Model file for the job. Use its own axes, mm. Face numbers are marked on the shaded views. A direction names the side the tool comes from. Give positions to 0.01 mm unless a question says otherwise; leave off trailing zeros. Loops run counter-clockwise (first coordinate to the right, second up) from the corner with the lowest first, then second, coordinate; pieces in that order, holes last. Notation, with made-up numbers: (33.25, -5.5) - (80.25, -5.5) arc R19 cw to (80.25, 17.5) - close; hole circle Ø3 at (37.5, -34.5). An arc over 180 degrees is marked (long way). Use a Markdown table: item, result.
Autodesk Inventor part; units mm, degrees
ref_plane "YZ Plane" through (0, 0, 0) normal (1, 0, 0) x (0, 1, 0)
ref_plane "XZ Plane" through (0, 0, 0) normal (0, 1, 0) x (-1, 0, 0)
ref_plane "XY Plane" through (0, 0, 0) normal (0, 0, 1) x (1, 0, 0)
sketch "Sketch1" plane through (0, 0, 0) normal (0, 1, 0) x (-1, 0, 0)
  circle A0 centre (0, 0) radius 72.5
  circle A1 centre (0, 0) radius 77.5
  circle A2 centre (0, 0) radius 53.5
  circle A3 centre (0, 0) radius 90 construction
  line L0 (0, 0) -> (-34.4415, 83.1492) construction
  circle A4 centre (-34.4415, 83.1492) radius 12
  line L1 (0, 154) -> (-32.5, 154)
  line L2 (-32.5, 154) -> (-32.5, 198)
  line L3 (-32.5, 198) -> (0, 198)
  line L4 (0, 198) -> (0, 154)
  line L5 (0, 140.825) -> (0, 198)
  line L6 (20, 74.8749) -> (-20, 74.8749)
  line L7 (-20, 74.8749) -> (-20, 154)
  line L8 (-20, 154) -> (20, 154)
  line L9 (20, 154) -> (20, 74.8749)
  line L10 (0, 0) -> (0, 198)
  line L11 (265, 193) -> (63.4449, 193)
  line L12 (63.4449, 193) -> (63.4449, 171)
  line L13 (63.4449, 171) -> (265, 171)
  line L14 (265, 171) -> (265, 193)
  line L15 (63.4449, 193) -> (0, 176)
  line L16 (63.4449, 171) -> (0, 154)
  line L17 (0, 154) -> (0, 176)
  arc A5 (-20, 106.132) -> (-41.3298, 99.779) centre (0, 0) ccw
  arc A6 (-41.3298, 99.779) -> (-51.0713, 76.2609) centre (-34.4415, 83.1492) ccw
  line L18 (-51.0713, 76.2609) -> (-45.4768, 62.7544)
  line L19 (-45.4768, 62.7544) -> (-20, 74.8749)
  line L20 (-20, 74.8749) -> (-20, 106.132)
  circle A7 centre (-34.4415, -83.1492) radius 12
  line L21 (0, 0) -> (-34.4415, -83.1492) construction
  line L22 (-45.4768, -62.7544) -> (-51.0713, -76.2609)
  arc A8 (-51.0713, -76.2609) -> (-34.4415, -101.1492) centre (-34.4415, -83.1492) ccw
  line L23 (-34.4415, -101.1492) -> (0, -101.1492)
  line L24 (0, -101.1492) -> (0, -77.5)
  line L25 (0, -77.5) -> (-45.4768, -62.7544)
  line L26 (265, 182) -> (164.2224, 182)
  line L27 (164.2224, 182) -> (164.2224, 171)
  line L28 (164.2224, 171) -> (265, 171)
  line L29 (265, 171) -> (265, 182)
  dimension "oDiaGasket" = 145
  dimension "oDiaOutside" = 155
  dimension "oDiaInside" = 107
  dimension "oHoledia" = 24
  dimension "oStemThick" = 40
  dimension "oAngleFirstBolt" = 22.5
  dimension "oKcircle" = 180
  dimension "oDiaTop" = 65
  dimension "oHeightTop" = 44
  dimension "oHandleLenght" = 265
  dimension "d10" = 5
  dimension "d11" = 15
  dimension "d13" = 6
  dimension "oCenterTop" = 198
  dimension "d32" = 22.5
  dimension "d33" = 6
sketch "Sketch2" plane through (0, 0, 0) normal (0, 1, 0) x (-1, 0, 0)
  circle A0 centre (0, 0) radius 77.5
  circle A1 centre (0, 0) radius 72.5
  circle A2 centre (0, 0) radius 53.5
extrude "Extrusion4" add sketch "Sketch2" along normal mid plane 56 contours A0 | A1 | A2
extrude "Extrusion5" add sketch "Sketch2" along normal mid plane 60 contours A1
extrude "Extrusion6" add sketch "Sketch1" along normal mid plane 40 contours A1 L10 L5 L8 L9 | L7 L1 L5 L10 A1
revolve "Revolution1" add sketch "Sketch1" angle 360 about axis through (0, 0, 0) along (0, 0, 1) contours L1 L2 L3 L4
extrude "Extrusion8" add sketch "Sketch1" along normal mid plane 15 contours A2 | A1 L18 A6 A5 L7 | L24 L23 A8 L22 A1
mirror "Mirror1" about plane through (0, 0, 0) normal (1, 0, 0) of "Extrusion8"
extrude "Extrusion9" add sketch "Sketch1" along normal mid plane 30 contours L4 L15 L12 L16 | L12 L11 L14 L26 L27 L13
chamfer "Chamfer1" distance 12 angle 45 4 edges at (-20, 20, 114.4374) (20, 20, 114.4374) (-20, -20, 114.4374) (20, -20, 114.4374)
equation "\"d32\" = oAngleFirstBolt"
equation "\"d33\" = d13"
equation "\"d25\" = oStemThick"
properties part number "BUTTERFLY VALVE MANUAL WAFER TYPE DN100" material "GG25"
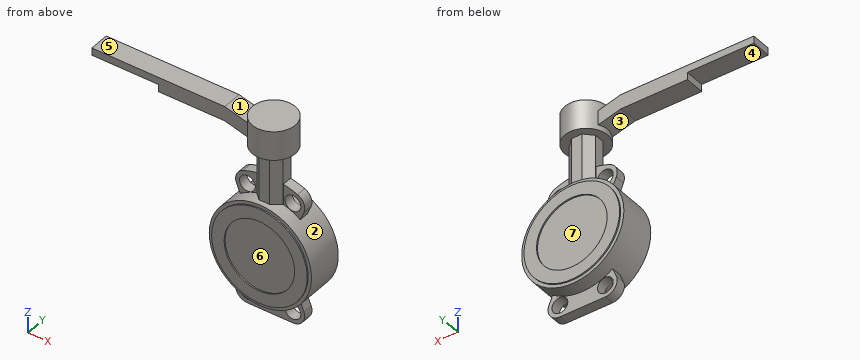
(1) Slice it at B-B, the plane z = 126.5. Write the cut outline in (x, y).
Computed:
| item | result |
|---|---|
| outline | (-20, -8) - (-8, -20) - (8, -20) - (20, -8) - (20, 8) - (8, 20) - (-8, 20) - (-20, 8) - close |
(2) Slice it at D-D, the plane z = 0. Write the cut outline in (x, y).
Computed:
| item | result |
|---|---|
| outline | (-77.5, -28) - (-72.5, -28) - (-72.5, -30) - (-53.5, -30) - (-53.5, -28) - (53.5, -28) - (53.5, -30) - (72.5, -30) - (72.5, -28) - (77.5, -28) - (77.5, 28) - (72.5, 28) - (72.5, 30) - (53.5, 30) - (53.5, 28) - (-53.5, 28) - (-53.5, 30) - (-72.5, 30) - (-72.5, 28) - (-77.5, 28) - close |
(3) Mould opens along X. For the marked faces 1, 2 and 3 say: pulls with the +X half, pulls with the -X half, needs draft (parallel to the pull), parting line crosses it, or undercut.
Computed:
| item | result |
|---|---|
| face 1 | undercut |
| face 2 | parting line crosses it |
| face 3 | pulls with the -X half |
(4) 3-axis set-ups, long thin cutter, end or side, ignore diameter. For the marked faces 4, 5, 6 and 7: which of +Z, -Z, +X, -X, +Y, -Y reach the whole face in a straight line?
Computed:
| item | result |
|---|---|
| face 4 | -Z, -X, +Y, -Y |
| face 5 | +Z, -X, +Y, -Y |
| face 6 | -Y |
| face 7 | +Y |
(5) Drill centre lines: probe 1 along Z at (x, y) = (0, 28.75); probe 2 along Y at (x, z) = (5, -18); probe 3 along Y at (x, z) = (-100, 175). Where is each one in solid material? Low to high. Write a range as [from, to].
Computed:
| item | result |
|---|---|
| probe 1 | [-72.5, -53.5], [53.5, 72.5], [154, 198] |
| probe 2 | [-28, 28] |
| probe 3 | [-15, 15] |
(6) Pin check, flat tips, straight feed: P1, Ø8, axis at y = -2, z = 95, coming from the -X side; P2, Ø1, axis at x = -67, y = -4.5, coming from the -Z side; P3, Ø24, axis at x = -210.5, y = 6, coming from the -Z side. Stop position of each tip, or through.
Computed:
| item | result |
|---|---|
| P1 | x = -50.64 |
| P2 | z = -39.8 |
| P3 | z = 182 |
(7) Slice it at C-C, the plane y = 0. Count the separate pieces of the cut face and the enclosed holes in it, plus the area to 3 significant figures.
Computed:
| item | result |
|---|---|
| separate pieces | 1 |
| enclosed holes | 4 |
| area | 31,900 mm² |
